Geometry check sheet. Reference: drawing and pictorial views, mm from the part's lowest x, y, z. Give positions to 0.01 mm unless a question says otherwise; leave off trailing zeros. Order: outer loops, then holes, each group sorted by start corner. A loop starts at its lowest first (then second) coordinate and runs counter-clockwise, first axis right, second up. Notation, with made-up numbers: M 11,55 L 61,55 A13 cw 61,63 Z; hole C 63.25,12 d7. An arc over 180 degrees is marked long. Answer as CSV lines item,"result".
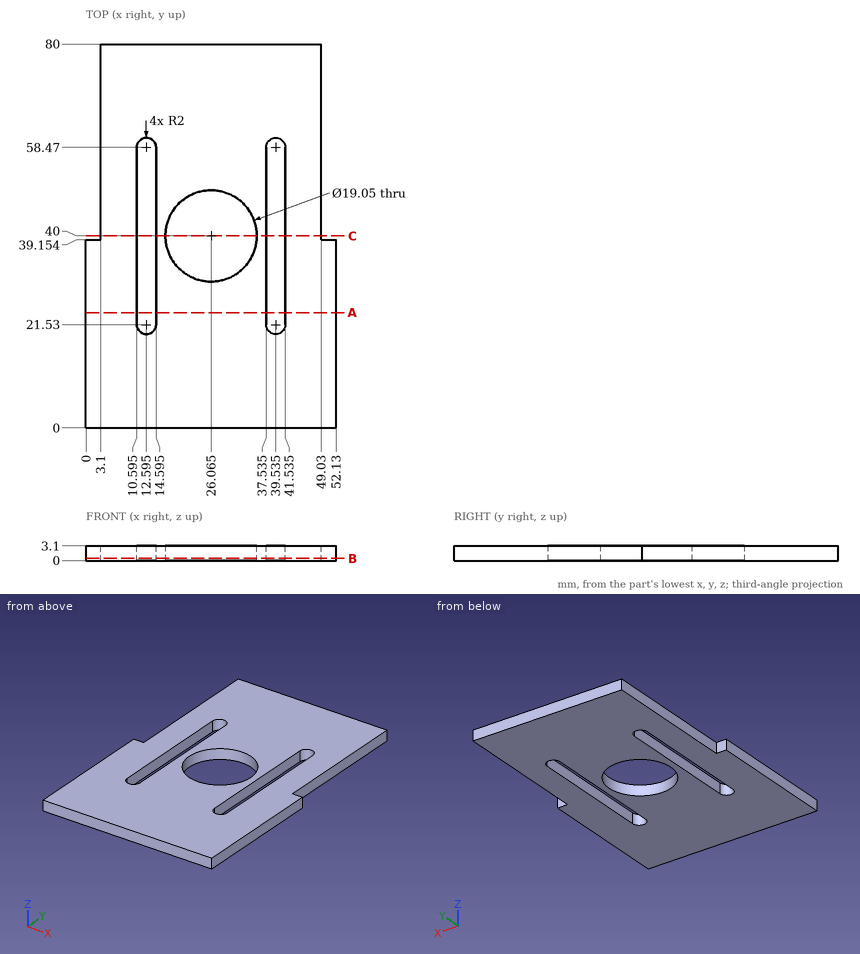
(1) Section check C-C on y = 40. Enter the section's corners in (x, z) (1 decimal).
The answers:
outline,"M 3.1,0 L 10.6,0 L 10.6,3.1 L 3.1,3.1 Z; M 14.6,0 L 16.5,0 L 16.5,3.1 L 14.6,3.1 Z; M 35.6,0 L 37.5,0 L 37.5,3.1 L 35.6,3.1 Z; M 41.5,0 L 49,0 L 49,3.1 L 41.5,3.1 Z"
(2) Gauge pin test, flat ends, axial feed: P1, Ø1.6, axis at y = 39.5, z = 2, coming from the -X side; P2, Ø0.9, axis at x = 2, z = 2, coming from the +Y side; P3, Ø0.9, axis at y = 53, z = 2, coming from the +X side. Record the tip position at first contact, or that the pin passes through.
The answers:
P1,"stops at x = 0"
P2,"stops at y = 39.15"
P3,"stops at x = 49.03"
(3) Material ranges on line 1 (X direction, y = 40, z = 0.95) (1 decimal); line 2 (X direction, y = 55.5, z = 2.9) (1 decimal); line 3 (Y direction, x = 49.5, z = 0.4), recorded low to high.
The answers:
line 1,"x = 3.1 to 10.6, 14.6 to 16.5, 35.6 to 37.5, 41.5 to 49"
line 2,"x = 3.1 to 10.6, 14.6 to 37.5, 41.5 to 49"
line 3,"y = 0 to 39.15"
(4) Section check A-A on y = 24. Enter the section's corners in (x, z) (1 decimal), then the cut area to 3 significant figures.
The answers:
outline,"M 0,0 L 10.6,0 L 10.6,3.1 L 0,3.1 Z; M 14.6,0 L 37.5,0 L 37.5,3.1 L 14.6,3.1 Z; M 41.5,0 L 52.1,0 L 52.1,3.1 L 41.5,3.1 Z"
area,"137 mm2"
(5) Section check B-B on z = 0.5. State how many separate pieces and enclosed holes the cut face has, then the cut area to 3 significant figures.
The answers:
separate pieces,"1"
enclosed holes,"3"
area,"3,310 mm2"
